Job drawing, mm, ordinate dimensions from the low corner. One solid piece. A direction names the side the tool comes from. Give positions to 0.01 mm unless a question says otherwise; leave off trailing zeros. Loops run counter-clockwise (first coordinate to the right, second up) from the corner with the lowest first, then second, coordinate; pieces in that order, holes last.
Item 1: Saw through at A-A on y = 5.25. Give the cut face in (x, z).
Item 2: Probe probe 1 along Y at (x, z) = (2, 32); probe 2 along Z at (x, y) = (21, 23.25). List the from-to ranges inside material, lowest first.
Item 3: Drop flat-ended pins along their axis: P1, Ø1.5, axis at x = 28.5, y = 4, coming from the +Z side; P2, Ø8, axis at x = 8, z = 25.5, coming from the +Y side; P3, Ø2.5, axis at y = 24, z = 11, coming from the +X side; P4, Ø1, axis at y = 10.5, z = 5.5, coming from the -X side. Give the stop position or say it passes through.
Item 4: Saw through at C-C on z = 24. Give the cut face in (x, y), plus the area to 3 significant figures.
Item 5: Saw through at D-D on x = 22. Give the cut face in (y, z), plus the area to 3 significant figures.
Item 6: Which spindle directions (+Z, -Z, +X, -X, +Y, -Y) get a long thin tool onto all of the face, cutting with end or side? Do the marked faces 1, 2 and 3. Say none if no direction does.
Item 7: Saw through at B-B on x = 16.5. Give the cut face in (y, z), plus the area to 4 significant figures.
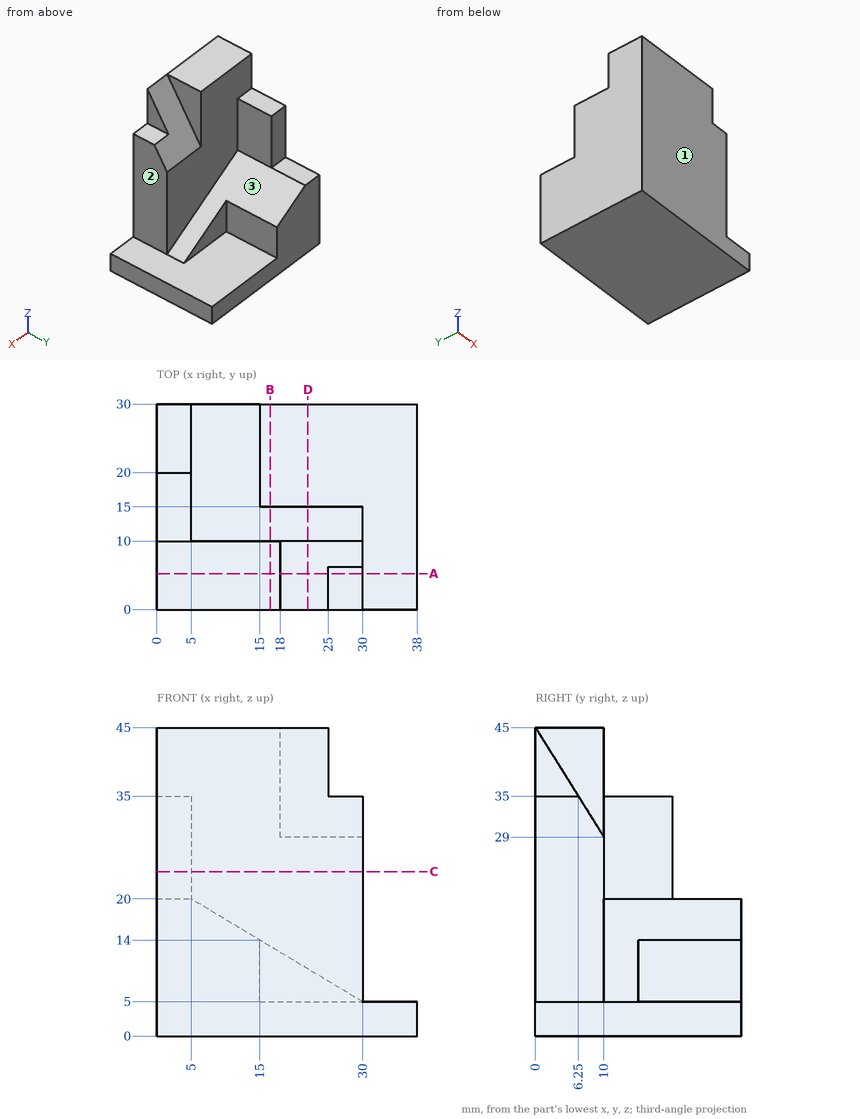
Results below:
1. outline: (0, 0) - (38, 0) - (38, 5) - (30, 5) - (30, 35) - (25, 35) - (25, 36.6) - (18, 36.6) - (18, 45) - (0, 45) - close
2. probe 1: y = 0 to 20
2. probe 2: z = 0 to 5
3. P1: stops at z = 35
3. P2: stops at y = 20
3. P3: stops at x = 15
3. P4: stops at x = 0
4. outline: (0, 0) - (30, 0) - (30, 10) - (5, 10) - (5, 20) - (0, 20) - close
4. area: 350 mm2
5. outline: (0, 0) - (30, 0) - (30, 5) - (15, 5) - (15, 9.8) - (10, 9.8) - (10, 29) - (0, 45) - close
5. area: 494 mm2
6. face 1: +Z, -Z, +X, -X, -Y
6. face 2: +Z, +X, +Y, -Y
6. face 3: +Z, +X, +Y
7. outline: (0, 0) - (30, 0) - (30, 5) - (15, 5) - (15, 13.1) - (10, 13.1) - (10, 45) - (0, 45) - close
7. area: 590.5 mm2
